Part model, mm, in its own coordinate system. Give positions to 0.01 mm unless a question says otherwise; leave off trailing zeros. Loops run counter-clockwise (first coordinate to the right, second up) from the corner with the lowest first, then second, coordinate; pieces in that order, holes last. Notation, with made-up numbers: M 83,-10 L 106,-10 A17 cw 106,-4 Z; hole C 52,-7 d8. An arc over 180 degrees is marked long. Answer in a Markdown table with one row per item.
from build123d import *

# Parameters (mm, degrees)
F0_W     = 5
F0_H     = 5
F1_DEPTH = 50
F2_R     = 4.99999


# Not quite as in the source:
# - a fillet or chamfer is up to 0.001 mm smaller than in the source, because OpenCascade refuses the exact size


with BuildPart() as f1:
    # F0 (on Top) → F1 (new body)
    with BuildSketch(Plane.XY):
        Rectangle(F0_W, F0_H)
    extrude(amount=F1_DEPTH)

    # F2 (radius 5 in the source; OpenCascade refuses exactly that, so slightly less here)
    f2_edges = [f1.edges().sort_by_distance(p)[0] for p in [
        (0, -2.5, 50),
    ]]
    fillet(f2_edges, radius=F2_R)


solid = f1.part
(1) Saw through at C-C (z = 46). Write the cut outline in (x, y), plus the area to 3 significant figures.
Recorded:
| item | result |
|---|---|
| outline | M -2.5,-2.4 L 2.5,-2.4 L 2.5,2.5 L -2.5,2.5 Z |
| area | 24.5 mm^2 |
(2) Drill centre lines: line 1 along Z through (x, y) = (1.6, 0.75); line 2 along Z through (x, y) = (-1.6, -0.55). Where is each one in solid material? Low to high.
Recorded:
| item | result |
|---|---|
| line 1 | z = 0 to 49.68 |
| line 2 | z = 0 to 48.96 |
(3) Saw through at B-B (y = -1). Write the cut outline in (x, z).
Recorded:
| item | result |
|---|---|
| outline | M -2.5,0 L 2.5,0 L 2.5,48.57 L -2.5,48.57 Z |
